```python
from build123d import *

# Parameters (mm, degrees)
F0_R      = 1.5
F1_DEPTH  = 15
F4_DEPTH  = 15
F5_R      = 2
F6_DEPTH  = 5
F7_R      = 2.85
F8_DEPTH  = 8.5
F9_R      = 2
F10_R     = 1.25
F11_DEPTH = 9
F13_DEPTH = 8
F14_R     = 2.85
F15_DEPTH = 5


with BuildPart() as f1:
    # F0 (on Front) → F1 (new body)
    with BuildSketch(Plane.XZ):
        with BuildLine():
            ThreePointArc((10.9369710195, -7.0272800513), (12.473584554, -3.6619241354), (13, 0))
            ThreePointArc((13, 0), (12.473584554, 3.6619241354), (10.9369710195, 7.0272800513))
            Line((10.9369710195, 7.0272800513), (10.9369710195, -7.0272800513))
        make_face()
        with BuildLine():
            ThreePointArc((10.9369710195, 7.0272800513), (12.473584554, 3.6619241354), (13, 0))
            ThreePointArc((13, 0), (12.473584554, -3.6619241354), (10.9369710195, -7.0272800513))
            Line((10.9369710195, -7.0272800513), (14.0475723892, -7.0272800513))
            Line((14.0475723892, -7.0272800513), (14.0475723892, 7.0272800513))
            Line((14.0475723892, 7.0272800513), (10.9369710195, 7.0272800513))
        make_face()
        with BuildLine():
            Line((10.9369710195, -7.0272800513), (10.9369710195, 7.0272800513))
            ThreePointArc((10.9369710195, 7.0272800513), (-13, 0), (10.9369710195, -7.0272800513))
        make_face()
        with Locations((0, -8)):
            Circle(F0_R, mode=Mode.SUBTRACT)
        with Locations((-8, 0)):
            Circle(F0_R, mode=Mode.SUBTRACT)
        with Locations((0, 8)):
            Circle(F0_R, mode=Mode.SUBTRACT)
    extrude(amount=F1_DEPTH)

    # F3 (on face) → F4 (cut)
    with BuildSketch(Plane.XZ.offset(15)):
        with BuildLine():
            ThreePointArc((11, 5), (10.7071067812, 5.7071067812), (10, 6))
            Line((10, 6), (10, 4))
            ThreePointArc((10, 4), (10.7071067812, 4.2928932188), (11, 5))
        make_face()
        with BuildLine():
            ThreePointArc((11, -5), (10.7071067812, -4.2928932188), (10, -4))
            Line((10, -4), (10, -6))
            ThreePointArc((10, -6), (10.7071067812, -5.7071067812), (11, -5))
        make_face()
        with BuildLine():
            Line((10, -6), (10, -4))
            ThreePointArc((10, -4), (9, -5), (10, -6))
        make_face()
        with BuildLine():
            Line((10, 4), (10, 6))
            ThreePointArc((10, 6), (9, 5), (10, 4))
        make_face()
    extrude(amount=-F4_DEPTH, mode=Mode.SUBTRACT)

    # F5 (on face) → F6 (cut)
    with BuildSketch(Plane.XZ):
        with Locations((10, 5)):
            Circle(F5_R)
        with Locations((10, -5)):
            Circle(F5_R)
    extrude(amount=F6_DEPTH, mode=Mode.SUBTRACT)

    # F7 (on face) → F8 (cut)
    with BuildSketch(Plane.XZ.offset(15)):
        with Locations((0, 8)):
            Circle(F7_R)
        with Locations((0, -8)):
            Circle(F7_R)
        with Locations((-8, 0)):
            Circle(F7_R)
    extrude(amount=-F8_DEPTH, mode=Mode.SUBTRACT)

    # F9
    f9_edges = [f1.edges().sort_by_distance(p)[0] for p in [
        (14.047572, -7.5, 7.02728),
        (14.047572, -7.5, -7.02728),
    ]]
    fillet(f9_edges, radius=F9_R)

    # F10 (on face) → F11 (cut)
    with BuildSketch(Plane.XZ):
        with Locations((9.2203840613, 9.2203840613)):
            Circle(F10_R)
    extrude(amount=F11_DEPTH, mode=Mode.SUBTRACT)

    # F12 (on face) → F13 (cut)
    with BuildSketch(Plane.XZ.offset(15)):
        with BuildLine():
            ThreePointArc((10.9369710195, 7.0272800513), (12.473584554, 3.6619241354), (13, 0))
            ThreePointArc((13, 0), (12.473584554, -3.6619241354), (10.9369710195, -7.0272800513))
            Line((10.9369710195, -7.0272800513), (12.0475723892, -7.0272800513))
            ThreePointArc((12.0475723892, -7.0272800513), (13.4617859516, -6.4414936136), (14.0475723892, -5.0272800513))
            Line((14.0475723892, -5.0272800513), (14.0475723892, 5.0272800513))
            ThreePointArc((14.0475723892, 5.0272800513), (13.4617859516, 6.4414936136), (12.0475723892, 7.0272800513))
            Line((12.0475723892, 7.0272800513), (10.9369710195, 7.0272800513))
        make_face()
    extrude(amount=-F13_DEPTH, mode=Mode.SUBTRACT)

    # F14 (on face) → F15 (cut)
    with BuildSketch(Plane.XZ.offset(15)):
        with BuildLine():
            Line((7.9317564177, -10.2998660248), (7.9317564177, 10.2998660248))
            ThreePointArc((7.9317564177, 10.2998660248), (-13, 0), (7.9317564177, -10.2998660248))
        make_face()
        with Locations((0, -8)):
            Circle(F14_R, mode=Mode.SUBTRACT)
        with Locations((-8, 0)):
            Circle(F14_R, mode=Mode.SUBTRACT)
        with Locations((0, 8)):
            Circle(F14_R, mode=Mode.SUBTRACT)
    extrude(amount=-F15_DEPTH, mode=Mode.SUBTRACT)


solid = f1.part
```
CAD build for the part. Positions are in the model's coordinates, mm. A direction names the side the tool comes from. Give positions to 0.01 mm unless a question says otherwise; leave off trailing zeros. Order: outer loops, then holes, each group sorted by start corner. A loop starts at its lowest first (then second) coordinate and runs counter-clockwise, first axis right, second up. Notation, with made-up numbers: M -14.75,60.25 L -10.75,60.25 A25 cw -10.75,99.25 Z; hole C 30,81 d1. An arc over 180 degrees is marked long. Put each result on its own line as item: value. Start each with the question number.
(1) Which spindle directions (+Z, -Z, +X, -X, +Y, -Y) get a long thin tool onto all of the face, cutting with end or side? Do faces 1 (the cylindrical face through (10, -2, 7)), 2 (the flat face through (-6.8, -6.5, -1.2)), 3 (the flat face through (-3, -10, 0)), 4 (the flat face through (11.5, -3.5, 7.027)). Say none if no direction does.
(2) Saw through at D-D, the plane x = -8.5. Write the cut outline in (y, z), then the cut area to 3 significant figures.
(3) Mould opens along X. For faces 5 (the cylindrical face through (8.4, -2.5, -6.2)), 6 (the flat face through (11.5, -3.5, -7.027)), 7 (the cylindrical face through (13.5, -3.5, 6.4)) say: +X half, -X half, draft (parallel to the pull), parting line (faces both ways), or undercut.
(4) Drill centre lines: line 1 along Z through (x, y) = (0, -1.75); line 2 along X through (y, z) = (-3.25, 0); line 3 along Z through (x, y) = (10.75, -7.75). Where is each one in solid material? Low to high.
(5) Flat gauge pins, fed straight in: pin 1 Ø5 at (x, z) = (-5.5, 3.5) entering from -Y; pin 2 Ø0.9 at (x, y) = (11.5, -2.5) entering from +Z; pin 3 Ø2.5 at (x, z) = (-8, 0) entering from +Y; pin 4 Ø1.2 at (x, z) = (10.5, 6) entering from +Y. Where does each tip first touch, or does it go through?
(6) Saw through at B-B, the plane y = -12.5. Write the cut outline in (x, z).
(7) Saw through at C-C, the plane z = -0.5. Write the cut outline in (x, y).
(8) Saw through at A-A, the plane x = 0. Write the cut outline in (y, z), then the cut area to 3 significant figures.
Check result:
1. face 1: +Y
1. face 2: -Y
1. face 3: +Z, -Z, -X, -Y
1. face 4: +Z, +X, +Y, -Y
2. outline: M -10,-9.84 L 0,-9.84 L 0,-1.41 L -6.5,-1.41 L -6.5,-2.81 L -10,-2.81 Z; M -10,2.81 L -6.5,2.81 L -6.5,1.41 L 0,1.41 L 0,9.84 L -10,9.84 Z
2. area: 159 mm2
3. face 5: undercut
3. face 6: draft
3. face 7: +X half
4. line 1: z = -13 to -9.5, -6.5 to 6.5, 9.5 to 13
4. line 2: x = -13 to -9.5, -6.5 to 14.05
4. line 3: z = -7.31 to -5.66, -4.34 to 4.34, 5.66 to 7.31
5. pin 1: stops at y = -10
5. pin 2: stops at z = 7.03
5. pin 3: passes through
5. pin 4: stops at y = -5
6. outline: M 7.93,-10.3 A13 ccw 7.93,10.3 Z; hole C 10,-5 d2; hole C 10,5 d2
7. outline: M -12.99,-10 L -10.81,-10 L -10.81,-6.5 L -9.41,-6.5 L -9.41,0 L -12.99,0 Z; M -6.59,-6.5 L -5.19,-6.5 L -5.19,-10 L 7.93,-10 L 7.93,-15 L 12.99,-15 L 12.99,-7 L 14.05,-7 L 14.05,0 L -6.59,0 Z
8. outline: M -10,-13 L 0,-13 L 0,-9.5 L -6.5,-9.5 L -6.5,-10.85 L -10,-10.85 Z; M -10,-5.15 L -6.5,-5.15 L -6.5,-6.5 L 0,-6.5 L 0,6.5 L -6.5,6.5 L -6.5,5.15 L -10,5.15 Z; M -10,10.85 L -6.5,10.85 L -6.5,9.5 L 0,9.5 L 0,13 L -10,13 Z
8. area: 181 mm2
